For this review, take the finished solid that the model builds, in its own axes (mm). A direction names the side the tool comes from. Round coordinates to 2 decimals unless told otherwise and drop trailing zeros. Order: outer loops, then holes, each group sorted by start corner. A loop starts at its lowest first (then second) coordinate and runs counter-clockwise, first axis right, second up. Notation, with made-up numbers: (23, 9.25) - (55, 9.25) arc R29 ccw to (55, 30.25) - close; hole circle Ø5 at (86, 64). An arc over 180 degrees is marked (long way). One line per item, written item: value.
```python
from build123d import *

# Parameters (mm, degrees)
SK_BRACKET_BASE_W     = 40
SK_BRACKET_BASE_H     = 3
BRACKET_BASE_DEPTH    = 40
SK_BRACKET_UPRIGHT_W  = 3
SK_BRACKET_UPRIGHT_H  = 40
BRACKET_UPRIGHT_DEPTH = 30
SK_CAMERA_W           = 22
SK_CAMERA_H           = 30
CAMERA_DEPTH          = 48.5


with BuildPart() as part:
    # SK_Bracket_Base → Bracket_Base (new, symmetric)
    with BuildSketch(Plane.XY):
        with Locations((-3, 1.5)):
            Rectangle(SK_BRACKET_BASE_W, SK_BRACKET_BASE_H)
    extrude(amount=BRACKET_BASE_DEPTH, both=True)

    # SK_Bracket_Upright → Bracket_Upright (add, symmetric)
    with BuildSketch(Plane.XY):
        with Locations((-12.5, 20)):
            Rectangle(SK_BRACKET_UPRIGHT_W, SK_BRACKET_UPRIGHT_H)
    extrude(amount=BRACKET_UPRIGHT_DEPTH, both=True)

    # SK_Camera → Camera (add, symmetric)
    with BuildSketch(Plane.XY):
        with Locations((0, 25)):
            Rectangle(SK_CAMERA_W, SK_CAMERA_H)
    extrude(amount=CAMERA_DEPTH, both=True)


solid = part.part
```
Item 1: Take a section at C-C (y = 11). Write out the cut boundary in (x, z), plus the area to 3 significant figures.
Returned:
outline: (-14, -30) - (-11, -30) - (-11, -48.5) - (11, -48.5) - (11, 48.5) - (-11, 48.5) - (-11, 30) - (-14, 30) - close
area: 2,310 mm^2
Item 2: Take a section at D-D (x = -13). Write out the cut boundary in (y, z).
Returned:
outline: (0, -40) - (3, -40) - (3, -30) - (40, -30) - (40, 30) - (3, 30) - (3, 40) - (0, 40) - close
Item 3: Wall thickness on line 1 (Y direction, x = -9, z = 32.5); line 2 (Y direction, x = 13, z = -10.5); line 3 (X direction, y = 30, z = -24.5): over which ranges is each line inside the solid? List them lowest first.
Returned:
line 1: 0 to 3, 10 to 40
line 2: 0 to 3
line 3: -14 to 11
Item 4: The part is to be moulded in two halves that separate along Y. For faces 5 (the flat face through (-3, 0, 1)), 6 (the flat face through (0, 10, 1)), 7 (the flat face through (0, 25, -48.5)), say which applies: +Y half, -Y half, draft (parallel to the pull), parting line (faces both ways), or undercut.
Returned:
face 5: -Y half
face 6: undercut
face 7: draft
Item 5: Machinability: for faces 1 (the flat face through (-13, 22, -30)), 2 (the flat face through (-13, 22, 30)), 3 (the flat face through (-3, 2, 40)), 4 (the flat face through (-11, 6, 0)), which of the approach directions +Z, -Z, +X, -X, +Y, -Y give a long, thin tool a straight path to every point of the face, cutting with its end or side? Answer none if there is none.
Returned:
face 1: -Z, -X, +Y
face 2: +Z, -X, +Y
face 3: +Z, +X, -X, -Y
face 4: +Z, -Z, +X
Item 6: Take a section at A-A (x = 9). Write out the cut boundary in (y, z), plus the area to 3 significant figures.
Returned:
outline: (0, -40) - (3, -40) - (3, 40) - (0, 40) - close; (10, -48.5) - (40, -48.5) - (40, 48.5) - (10, 48.5) - close
area: 3,150 mm^2
Item 7: For P1, Ø4, axis at y = 22.5, z = -10.5, coming from the +X side; P2, Ø6, axis at y = 16.5, z = 29, coming from the -X side; P3, Ø5.5, axis at y = 18.5, z = -38, coming from the -X side, all flat-tipped, find the tip position at first contact; note any pin that passes through.
Returned:
P1: x = 11
P2: x = -14
P3: x = -11
Item 8: Take a section at B-B (z = 33). Write out the cut boundary in (x, y), plus the area to 3 significant figures.
Returned:
outline: (-23, 0) - (17, 0) - (17, 3) - (-23, 3) - close; (-11, 10) - (11, 10) - (11, 40) - (-11, 40) - close
area: 780 mm^2
